For this review, take the finished solid that the model builds, in its own axes (mm). A direction names the side the tool comes from. Coordinates: 2 decimals unless noted, no trailing zeros. Write each loop counter-clockwise with the first axis right and the second up, starting at its lowest first coordinate (ties: lowest second). Pieces come first, ordered by that corner, then holes. Notation, with made-up numbers: (-24.5, 20.25) - (3.5, 20.25) arc R29 ccw to (3.5, 54.25) - close; hole circle Ø5 at (-21, -13). An arc over 180 degrees is marked (long way). Write each question's results on one line, items separated by ' | '.
from build123d import *

# Parameters (mm, degrees)
BOSS_EXTRU_1_DEPTH      = 9
ESQUISSE2_W             = 19.623971562
ESQUISSE2_H             = 15.534154535
ESQUISSE2_R             = 3
ENL_V_MAT_EXTRU_1_DEPTH = 3
ENL_V_START             = -4
ESQUISSE3_W             = 11.267201257
ESQUISSE3_H             = 13.961169169
ESQUISSE3_R             = 3
ENL_V_MAT_EXTRU_2_DEPTH = 4
CHANFREIN1_SIZE         = 4
CHANFREIN1_SIZE_2       = 2.499477408


with BuildPart() as part:
    # Esquisse1 → Boss.-Extru.1 (new body)
    with BuildSketch(Plane.XY):
        Polygon((4.041451884, 0), (2.020725942, 3.5), (-2.020725942, 3.5), (-4.041451884, 0), (-2.020725942, -3.5), (2.020725942, -3.5), align=None)
    extrude(amount=BOSS_EXTRU_1_DEPTH)

    # Esquisse2 → Enlèv. mat.-Extru.1 (cut)
    with BuildSketch(Plane.XY.offset(9)):
        with Locations((0.327116653, -1.544441398)):
            Rectangle(ESQUISSE2_W, ESQUISSE2_H)
        Circle(ESQUISSE2_R, mode=Mode.SUBTRACT)
    extrude(amount=-ENL_V_MAT_EXTRU_1_DEPTH, mode=Mode.SUBTRACT)

    # Esquisse3 → Enlèv. mat.-Extru.2 (cut)
    with BuildSketch(Plane(origin=(0, 0, 0), x_dir=(-1, 0, 0), z_dir=(0, 0, -1)).offset(ENL_V_START)):
        with Locations((0.009770186, 0.039262349)):
            Rectangle(ESQUISSE3_W, ESQUISSE3_H)
        with Locations(Location((0, 0, 0), (0, 0, 180))):
            Circle(ESQUISSE3_R, mode=Mode.SUBTRACT)
    extrude(amount=ENL_V_MAT_EXTRU_2_DEPTH, mode=Mode.SUBTRACT)

    # Chanfrein1
    # the kernel refuses this chamfer: 4, 2.499477408 mm, written as the material it takes off along each edge
    with BuildSketch(Plane(origin=(0, 0, 0), x_dir=(1, 0, 0), z_dir=(0, 1, 0))) as chanfrein1_piece_1_section:
        Polygon((3, -CHANFREIN1_SIZE), (3 - CHANFREIN1_SIZE_2, 0), (3, 0), align=None)
    chanfrein1_piece_1 = revolve(axis=Axis((0, 0, 0), (0, 0, -1)), mode=Mode.PRIVATE)
    chanfrein1_piece_1 = split(chanfrein1_piece_1, bisect_by=Plane(origin=(-1.744026904, 0, 4), z_dir=(0, 0, -1)), keep=Keep.TOP, mode=Mode.PRIVATE)
    add(chanfrein1_piece_1, mode=Mode.SUBTRACT)

    # Esquisse4 → Enlèvement de matière-Révolution1 (revolve, cut)
    with BuildSketch(Plane(origin=(0, 0, 0), x_dir=(1, 0, 0), z_dir=(0, 1, 0))):
        Polygon((0, -9), (1, -9), (1, -6.922694464), (0.15, 0), (0, 0), align=None)
    revolve(axis=Axis((0, 0, 10.381605157), (0, 0, -1)), mode=Mode.SUBTRACT)


solid = part.part
Q1. Take a section at A-A on x = 0. State the section outline as (y, z) points, plus the area to 3 significant figures.
Results found:
outline: (-3.5, 4) - (-3, 4) - (-0.5, 0) - (-0.15, 0) - (-1, 6.92) - (-1, 9) - (-3, 9) - (-3, 6) - (-3.5, 6) - close; (0.15, 0) - (0.5, 0) - (3, 4) - (3.5, 4) - (3.5, 6) - (3, 6) - (3, 9) - (1, 9) - (1, 6.92) - close | area: 33.9 mm2
Q2. Take a section at D-D on z = 1.75. State the section outline as (x, y) points.
Results found:
outline: circle Ø3.19 at (0, 0); hole circle Ø0.73 at (0, 0)
Q3. Take a section at B-B on z = 7.25. State the section outline as (x, y) points.
Results found:
outline: circle Ø6 at (0, 0); hole circle Ø2 at (0, 0)
Q4. Wall thickness on line 1 along Y through (x, z) = (0, 8.15); line 2 along Z through (x, y) = (-2, 2.5); line 3 along X through (y, z) = (0.5, 5.5): over which ranges is each line inside the solid? List them lowest first. Write a range as from..to.
Results found:
line 1: -3..-1, 1..3 | line 2: 4..6 | line 3: -3.75..-0.66, 0.66..3.75
Q5. For faces 1 (the face through (1, 3, 4)), 2 (the face through (-3.045, -1.726, 4.986)), 3 (the face through (0, 1, 8)), list the 3-axis set-ups (+Z, -Z, +X, -X, +Y, -Y) from which the entire face can be reached by the end or side of a thin tool; tool diameter is ignored.
Results found:
face 1: -Z | face 2: +Z, -Z, -X, -Y | face 3: +Z
Q6. Mouldability with a two-part tool opening along X and no side actions: class faces 4 (the face through (-3, 1.8, 5)), 5 (the face through (-0.123, 0.556, 3.413)), 6 (the face through (-1, 1, 9)) as pulls with the +X half, pulls with the -X half, needs draft (parallel to the pull), parting line crosses it, or undercut.
Results found:
face 4: pulls with the -X half | face 5: undercut | face 6: needs draft
Q7. For pin 1 (1.2 mm diameter, centred on x = 0, y = 0, fed in from -Z); pin 2 (4 mm diameter, centred on y = -2, z = 7.5, fed in from +X), all flat-tipped, find the tip position at first contact; note any pin that passes through.
Results found:
pin 1: z = 0 | pin 2: x = 3.65
Q8. Take a section at C-C on x = -3.5. State the section outline as (y, z) points.
Results found:
outline: (-0.94, 4) - (0.94, 4) - (0.94, 6) - (-0.94, 6) - close
